Input: part model. Units: mm. Frame: model coordinates. Face numbers are marked on the shaded views. Give positions to 0.01 mm unless a question says otherwise; leave off trailing zeros. Write each loop counter-clockwise with the first axis right and the second up, starting at its lowest first coordinate (ties: lowest second). Pieces come first, ordered by that corner, then holes.
```python
from build123d import *

# Parameters (mm, degrees)
F0_W      = 5.3958347999
F0_H      = 30.1875006407
F0_W_2    = 3.7958348403
F0_H_2    = 28.5875006812
F1_DEPTH  = 10
F4_DEPTH  = 6.7
F3_W      = 2.0448579453
F3_H      = 6.6219959408
F5_DEPTH  = 31.8
F6_DEPTH  = 6.5
F3_W_2    = 5.3958347999
F3_H_2    = 1.2
F7_DEPTH  = 6.9
F8_DEPTH  = 30.1
F10_DEPTH = 1.42
F9_W      = 3.3958347049
F9_H      = 3.9405850694
F11_DEPTH = 1.3


with BuildPart() as f1:
    # F0 (on Top) → F1 (new body)
    with BuildSketch(Plane.XY):
        with Locations((-2.6979173999, 15.0937503204)):
            Rectangle(F0_W, F0_H)
        with Locations((-2.6979173999, 15.0937503204)):
            Rectangle(F0_W_2, F0_H_2, mode=Mode.SUBTRACT)
    extrude(amount=F1_DEPTH)

    # F2 (on face) → F4 (cut)
    with BuildSketch(Plane.YZ):
        Polygon((28.6875006277, 1.500000013), (27.6875006966, 2.4999999441), (18.2672608644, 2.4999999441), (16.5937503204, 0), (30.1875006407, 0), align=None)
        Polygon((2.4999999441, 2.4999999441), (1.500000013, 1.500000013), (0, 0), (13.5937503204, 0), (11.9336228818, 2.4999999441), align=None)
    extrude(amount=-F4_DEPTH, mode=Mode.SUBTRACT)

    # F3 (on face) → F5 (cut)
    with BuildSketch(Plane(origin=(0, 30.1875006407, 0), x_dir=(-1, 0, 0), z_dir=(0, 1, 0))):
        with Locations((2.6979173999, 3.3109979704)):
            Rectangle(F3_W, F3_H)
    extrude(amount=-F5_DEPTH, mode=Mode.SUBTRACT)

    # F2 (on face) → F6 (cut)
    with BuildSketch(Plane.YZ):
        Polygon((18.2681400329, 7.5000000559), (27.6875006966, 7.5000000559), (28.6875006277, 8.499999987), (28.6875006277, 10), (16.5937503204, 10), align=None)
        Polygon((1.500000013, 10), (1.500000013, 8.499999987), (2.4999999441, 7.5000000559), (11.9306277484, 7.5000000559), (13.5937503204, 10), align=None)
    extrude(amount=-F6_DEPTH, mode=Mode.SUBTRACT)

    # F3 (on face) → F7 (join)
    with BuildSketch(Plane(origin=(0, 30.1875006407, 0), x_dir=(-1, 0, 0), z_dir=(0, 1, 0))):
        with Locations((2.6979173999, 9.4)):
            Rectangle(F3_W_2, F3_H_2)
    extrude(amount=-F7_DEPTH)

    # F3 (on face) → F8 (join)
    with BuildSketch(Plane(origin=(0, 30.1875006407, 0), x_dir=(-1, 0, 0), z_dir=(0, 1, 0))):
        with Locations((2.6979173999, 9.4)):
            Rectangle(F3_W_2, F3_H_2)
    extrude(amount=-F8_DEPTH)

    # F9 (on face) → F10 (cut)
    with BuildSketch(Plane.XY.offset(10)):
        Polygon((-5.3958347999, 1.0000000475), (-4.3958347524, 1.0000000475), (-4.3958347524, 11.153165251), (-4.3958347524, 15.0937503204), (-4.3958347524, 19.0343353897), (-4.3958347524, 29.1875005933), (-5.3958347999, 29.1875005933), align=None)
        Polygon((-1.0000000475, 11.153165251), (-1.0000000475, 1.0000000475), (0, 1.0000000475), (0, 29.1875005933), (-1.0000000475, 29.1875005933), (-1.0000000475, 19.0343353897), (-1.0000000475, 15.0937503204), align=None)
    extrude(amount=-F10_DEPTH, mode=Mode.SUBTRACT)

    # F9 (on face) → F11 (cut)
    with BuildSketch(Plane.XY.offset(10)):
        with Locations((-2.6979173999, 13.1234577857)):
            Rectangle(F9_W, F9_H)
        with Locations((-2.6979173999, 17.0640428551)):
            Rectangle(F9_W, F9_H)
    extrude(amount=-F11_DEPTH, mode=Mode.SUBTRACT)


solid = f1.part
```
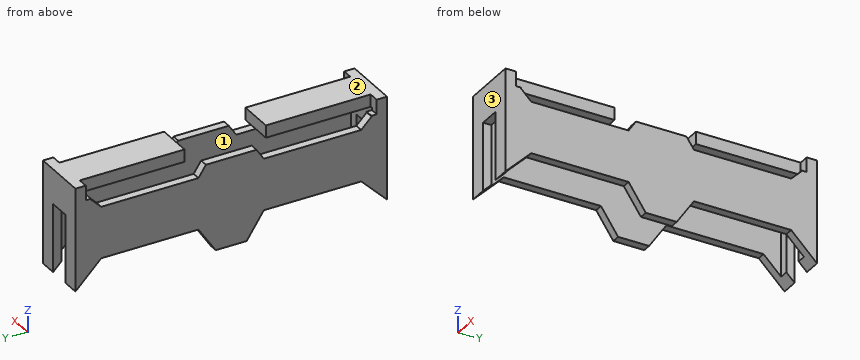
Q1. Pin query (flat end, axial travel): pin 1 (2 mm diameter, centred on x = -1, y = 21.5, fed in from -Z). Return the tip coordinate at first contact, or that it passes through.
Q2. Section D-D, the plane z = 1.75. Give the number of separate pieces and of enclosed holes in the cut face, then the cut area to 3 significant figures.
Q3. Section B-B, the plane x = -3.3. Return the cut outline in (y, z).
Q4. Section C-C, the plane z = 3.75. Return the cut outline in (x, y), then the cut area to 3 significant figures.
Q5. Mould query, pull axis Y, two halves, no side actions, for the marked faces 1, 2 and 3. Classes: +Y half, -Y half, draft (parallel to the pull), parting line (faces both ways), or undercut.
Q6. Material intervals for line 1 along Y through (x, z) = (-4.5, 1.25); line 2 along X through (y, z) = (2, 6); line 3 along Y through (x, z) = (-0.25, 9.5), sorted ascending.
Q7. Section A-A, the plane y = 27. Return the cut outline in (x, z), then the cut area to 3 significant figures.
Solutions:
1. pin 1: stops at z = 2.5
2. separate pieces: 6
2. enclosed holes: 0
2. area: 16.9 mm2
3. outline: (0, 6.62) - (0.8, 6.62) - (0.8, 8.8) - (11.15, 8.8) - (11.15, 10) - (0, 10) - close; (19.03, 8.8) - (29.39, 8.8) - (29.39, 6.62) - (30.19, 6.62) - (30.19, 10) - (19.03, 10) - close
4. outline: (-5.4, 0) - (-3.72, 0) - (-3.72, 0.8) - (-4.6, 0.8) - (-4.6, 29.39) - (-3.72, 29.39) - (-3.72, 30.19) - (-5.4, 30.19) - close; (-1.68, 0) - (0, 0) - (0, 30.19) - (-1.68, 30.19) - (-1.68, 29.39) - (-0.8, 29.39) - (-0.8, 0.8) - (-1.68, 0.8) - close
4. area: 51.1 mm2
5. face 1: undercut
5. face 2: draft
5. face 3: -Y half
6. line 1: y = 0 to 0.8, 29.39 to 30.19
6. line 2: x = -5.4 to -4.6, -0.8 to 0
6. line 3: y = 0 to 1, 29.19 to 30.19
7. outline: (-5.4, 2.5) - (-4.6, 2.5) - (-4.6, 7.5) - (-5.4, 7.5) - close; (-4.4, 8.8) - (-1, 8.8) - (-1, 10) - (-4.4, 10) - close; (-0.8, 2.5) - (0, 2.5) - (0, 7.5) - (-0.8, 7.5) - close
7. area: 12.1 mm2
